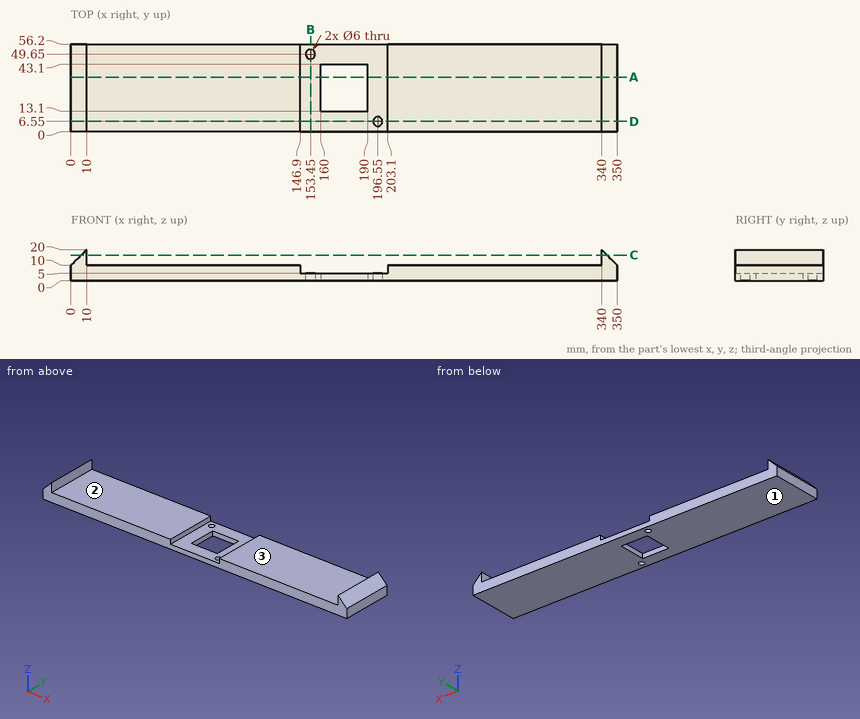
Could you check a few things on this drawing? It's one solid part, dimensions in mm from its lowest x, y, z. Give positions to 0.01 mm unless a question says otherwise; leave off trailing zeros. Order: outer loops, then holes, each group sorted by start corner. A loop starts at its lowest first (then second) coordinate and runs counter-clockwise, first axis right, second up. Notation, with made-up numbers: (76, -21.5) - (104, -21.5) arc R13 ccw to (104, 1.5) - close; hole circle Ø3 at (78.5, -8.75). An arc over 180 degrees is marked (long way). One line per item, written item: value. Start each with the question number.
1. Imagine slicing it at B-B on x = 153.45. List the corners of the cut face in (y, z) for me, plus the area to 3 significant figures.
2. Imagine slicing it at C-C on z = 16.5. List the corners of the cut face in (x, y) for me, plus the area to 3 significant figures.
3. Imagine slicing it at A-A on y = 35. List the corners of the cut face in (x, z) for me.
4. For P1, Ø8, axis at y = 41, z = 17, coming from the +X side; P2, Ø3, axis at y = 35.5, z = 15, coming from the -X side; P3, Ø17, axis at x = 74.5, y = 33, coming from the +Z side; P4, Ø8, axis at x = 209, z = 17, coming from the +Y side, each with a flat end and sliding along its axis, tell me the tip position at first contact or that it passes through.
5. If I drill on probe 1 along X at (y, z) = (50, 3); probe 2 along Y at (x, z) = (196.55, 1.35); probe 3 along X at (y, z) = (21, 6.75), over which ranges is the centre line in solid material (lowest first)?
6. Thinking about a two-plate mould opening in X: for the marked faces 1, 2 and 3, which applies, +X half, -X half, draft (parallel to the pull), parting line (faces both ways), or undercut?
7. Imagine slicing it at D-D on y = 6.55. List the corners of the cut face in (x, z) for me, plus the area to 3 significant figures.
Values:
1. outline: (0, 0) - (46.65, 0) - (46.65, 5) - (0, 5) - close; (52.65, 0) - (56.2, 0) - (56.2, 5) - (52.65, 5) - close
1. area: 251 mm²
2. outline: (6.5, 0) - (10, 0) - (10, 56.2) - (6.5, 56.2) - close; (340, 0) - (343.5, 0) - (343.5, 56.2) - (340, 56.2) - close
2. area: 393 mm²
3. outline: (0, 0) - (160, 0) - (160, 5) - (146.9, 5) - (146.9, 10) - (10, 10) - (10, 20) - (0, 10) - close; (190, 0) - (350, 0) - (350, 10) - (340, 20) - (340, 10) - (203.1, 10) - (203.1, 5) - (190, 5) - close
4. P1: x = 347
4. P2: x = 3.5
4. P3: z = 10
4. P4: through
5. probe 1: 0 to 150.47, 156.43 to 350
5. probe 2: 0 to 3.55, 9.55 to 56.2
5. probe 3: 0 to 146.9, 203.1 to 350
6. face 1: draft
6. face 2: undercut
6. face 3: undercut
7. outline: (0, 0) - (193.55, 0) - (193.55, 5) - (146.9, 5) - (146.9, 10) - (10, 10) - (10, 20) - (0, 10) - close; (199.55, 0) - (350, 0) - (350, 10) - (340, 20) - (340, 10) - (203.1, 10) - (203.1, 5) - (199.55, 5) - close
7. area: 3,290 mm²
